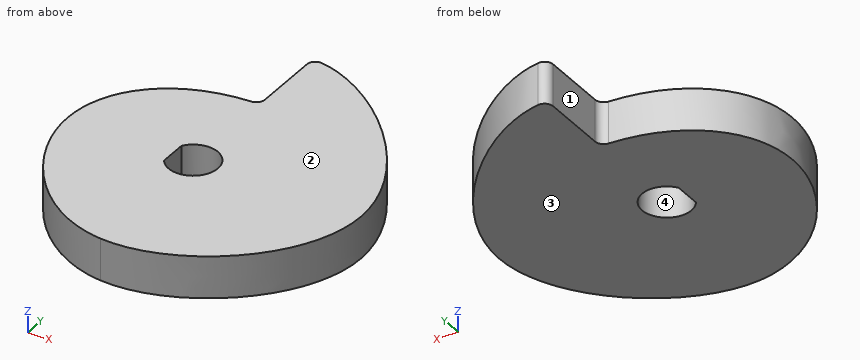
from build123d import *

# Parameters (mm, degrees)
F1_DEPTH = 5
F3_DEPTH = 5


with BuildPart() as f1:
    # F0 (on Top) → F1 (new body)
    with BuildSketch(Plane.XY):
        with BuildLine():
            ThreePointArc((1.1420704693, 22.4149806807), (0.3450459823, 22.180792868), (0, 21.4251241346))
            Line((0, 21.4251241346), (0, 13.4793751215))
            ThreePointArc((0, 13.4793751215), (-0.2783323598, 12.7871354108), (-0.9583916341, 12.4802411245))
            add(Edge.make_bspline(
                [(-0.9583916341, 12.4802411245), (-9.7677869501, 12.1133788767), (-20.8879182433, 0.572881244), (-8.3742030553, -16.6290905544), (0, -17.5)],
                knots=[0.0076786773, 0.0076786773, 0.0076786773, 0.0076786773, 0.2224792249, 0.4641987518, 0.4641987518, 0.4641987518, 0.4641987518], degree=3))
            add(Edge.make_bspline(
                [(0, -17.5), (8.9920428291, -18.4351642161), (31.1411413145, -1.2068050011), (8.7240631606, 21.3267651565), (1.1420704693, 22.4149806807)],
                knots=[0.4641987518, 0.4641987518, 0.4641987518, 0.4641987518, 0.7237520877, 0.9864457327, 0.9864457327, 0.9864457327, 0.9864457327], degree=3))
        make_face()
    extrude(amount=F1_DEPTH)

    # F2 (on face) → F3 (cut)
    with BuildSketch(Plane.XY.offset(5)):
        with BuildLine():
            ThreePointArc((-2.45, -1.6431676725), (2.95, 0), (-2.45, 1.6431676725))
            Line((-2.45, 1.6431676725), (-2.45, -1.6431676725))
        make_face()
    extrude(amount=-F3_DEPTH, mode=Mode.SUBTRACT)


solid = f1.part
Read the model definition and answer for the solid it produces. Units are mm, in the model's axes. Face numbers are marked on the shaded views. A direction names the side the tool comes from. Round coordinates to 2 decimals unless told otherwise and drop trailing zeros. One line per question, with ' | ' between items. Start each with the question number.
1. For the marked faces 1 and 2, determine the directions among +Z, -Z, +X, -X, +Y, -Y from which every point of the face is accessible in a straight line to the end or side of a thin tool.
2. For a pull along Y with two mould halves and no side action, classify the marked faces 3 and 4 as +Y half, -Y half, draft (parallel to the pull), parting line (faces both ways), or undercut.
3. Each of these flat-tipped pins is pushed along its axis until it touches: pin 1 (3 mm diameter, centred on y = -6.5, z = 3.5, fed in from +X); pin 2 (3 mm diameter, centred on y = 13.5, z = 3.5, fed in from +X). Where does it stop, or does it pass through?
Filled in:
1) face 1: +Z, -Z, -X, +Y | face 2: +Z, +X, -X, +Y, -Y
2) face 3: draft | face 4: undercut
3) pin 1: x = 19.07 | pin 2: x = 15.47
